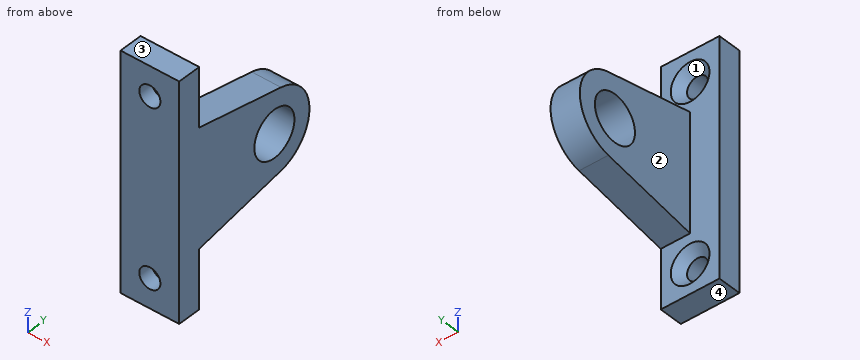
from build123d import *

# Parameters (mm, degrees)
SKETCH_1_R                = 4
EXTRUDE_1_DEPTH           = 5
SKETCH_2_W                = 5
SKETCH_2_H                = 40
EXTRUDE_2_DEPTH           = 4
HOLE_WIZARD_1_D           = 3.6
HOLE_WIZARD_1_CSINK_D     = 6.6
HOLE_WIZARD_1_CSINK_ANGLE = 90


with BuildPart() as part:
    # 草图1 → 凸台-拉伸1 (new body)
    with BuildSketch(Plane(origin=(0, 0, 0), x_dir=(0, 0, -1), z_dir=(1, 0, 0))):
        with BuildLine():
            Line((-6.875049265, 20.31669951), (-10, 4))
            Line((-10, 4), (-20, 4))
            Line((-20, 4), (-20, 0))
            Line((-20, 0), (20, 0))
            Line((20, 0), (20, 4))
            Line((20, 4), (10, 4))
            Line((10, 4), (6.875049265, 20.31669951))
            ThreePointArc((6.875049265, 20.31669951), (0, 26), (-6.875049265, 20.31669951))
        make_face()
        with Locations((0, 19)):
            Circle(SKETCH_1_R, mode=Mode.SUBTRACT)
    extrude(amount=EXTRUDE_1_DEPTH)

    # 草图2 → 凸台-拉伸2 (add)
    with BuildSketch(Plane(origin=(0, 4, 0), x_dir=(1, 0, 0), z_dir=(0, 1, 0))):
        with Locations((-2.5, 0)):
            Rectangle(SKETCH_2_W, SKETCH_2_H)
    extrude(amount=-EXTRUDE_2_DEPTH)

    # 打孔尺寸(%根据十字)槽半沉头木螺钉的类型1 (through all)
    with Locations(Plane(origin=(0, 4, 0), x_dir=(1, 0, 0), z_dir=(0, 1, 0))):
        with Locations((0, 15), (0, -15)):
            CounterSinkHole(HOLE_WIZARD_1_D / 2, HOLE_WIZARD_1_CSINK_D / 2, counter_sink_angle=HOLE_WIZARD_1_CSINK_ANGLE)


solid = part.part
Could you check a few things on this model? Use its own coordinates, in mm. Face numbers are marked on the shaded views. Give positions to 0.01 mm unless a question says otherwise; leave off trailing zeros. Order: outer loops, then holes, each group sorted by start corner. A loop starts at its lowest first (then second) coordinate and runs counter-clockwise, first axis right, second up.
Item 1: If we section it at C-C, the plane z = 0: Write out the boundary of the cut face in (x, y), plus the area to 3 significant figures.
Item 2: If we section it at D-D, the plane x = -4.5: Write out the boundary of the cut face in (y, z).
Item 3: If we section it at B-B, the plane y = 19.5: Write out the boundary of the cut face in (x, z), plus the area to 3 significant figures.
Item 4: If we section it at A-A, the plane z = 15: Write out the boundary of the cut face in (x, y), plus the area to 4 significant figures.
Item 5: I'm going to push flat-ended pins straight in: pin 1 (10 mm diameter, centred on y = 13.5, z = 2, fed in from -X); pin 2 (6 mm diameter, centred on x = 0, z = 15, fed in from +Y); pin 3 (6 mm diameter, centred on x = -3.5, z = -12.5, fed in from +Y). Where does each tip first touch, or does it pass through?
Item 6: If we mould it in two halves opening along Z, with no side actions, what happens to the marked faces 1, 2, 3 and 4? For each: pulls with the +Z half, pulls with the -Z half, needs draft (parallel to the pull), parting line crosses it, or undercut.
Item 7: I need wall thicknesses on line 1 (Z direction, x = 0, y = 0.8); line 2 (Y direction, x = 2.4, z = 0); line 3 (X direction, y = 1.8, z = -15). Which ranges of each line are inside material? Lowest first, please.
Values:
1. outline: (-5, 0) - (5, 0) - (5, 15) - (0, 15) - (0, 4) - (-5, 4) - close; (0, 23) - (5, 23) - (5, 26) - (0, 26) - close
1. area: 110 mm2
2. outline: (0, -20) - (4, -20) - (4, 20) - (0, 20) - close
3. outline: (0, -7.03) - (5, -7.03) - (5, -3.97) - (0, -3.97) - close; (0, 3.97) - (5, 3.97) - (5, 7.03) - (0, 7.03) - close
3. area: 30.6 mm2
4. outline: (-5, 0) - (-1.8, 0) - (-1.8, 2.5) - (-3.3, 4) - (-5, 4) - close; (1.8, 0) - (5, 0) - (5, 4) - (3.3, 4) - (1.8, 2.5) - close
4. area: 23.35 mm2
5. pin 1: stops at x = 0
5. pin 2: stops at y = 3.7
5. pin 3: stops at y = 4
6. face 1: undercut
6. face 2: needs draft
6. face 3: pulls with the +Z half
6. face 4: pulls with the -Z half
7. line 1: z = -20 to -16.8, -13.2 to 13.2, 16.8 to 20
7. line 2: y = 0 to 15, 23 to 26
7. line 3: x = -5 to -1.8, 1.8 to 5
